The model under review builds one solid part; all positions refer to its coordinate system, in mm. A direction names the side the tool comes from. Coordinates: 2 decimals unless noted, no trailing zeros. Order: outer loops, then holes, each group sorted by start corner. A loop starts at its lowest first (then second) coordinate and runs counter-clockwise, first axis right, second up. Notation, with made-up numbers: M -31.75,26.5 L -1.75,26.5 A19 ccw -1.75,55.5 Z; hole C -11.75,2.25 d1. An arc over 180 degrees is marked long. Answer as CSV lines item,"result". Start each with the question number.
Q1. Machinability: for faces 5 (the face through (-17.691, -13, 6)), 6 (the face through (1, 0, 2)), which of the approach directions +Z, -Z, +X, -X, +Y, -Y give a long, thin tool a straight path to every point of the face, cutting with its end or side? Answer none if there is none.
Q2. Consider section B-B on z = 25. Write out the cut boundary in (x, y), and give its area (3 significant figures).
Q3. The part is to be moulded in two halves that separate along X. For faces 1 (the face through (-3, -13, -20.358)), 2 (the face through (1, -13, -42.939)), 3 (the face through (-46.495, -13, 0)), 4 (the face through (36.716, -13, 25)), say which applies: +X half, -X half, draft (parallel to the pull), parting line (faces both ways), or undercut.
Q4. Consider section D-D on x = -27. Write out the cut boundary in (y, z), and give its area (3 significant figures).
Q5. Consider section C-C on y = -21. Write out the cut boundary in (x, z), and give its area (3 significant figures).
Q6. Wall thickness on L1, parallel to Z at x = 17, y = -19.5; L2, parallel to Z at x = 29.5, y = -4.75; L3, parallel to X at y = -10.75, z = 26: over which ranges is each line inside the solid? List them lowest first. Write a range as [from, to].
Q7. Consider section A-A on x = -5. Write out the cut boundary in (y, z), and give its area (3 significant figures).
Q8. For P1, Ø1, axis at x = -13, z = -11.5, coming from the +Y side, flat-tipped, find the tip position at first contact; note if it passes through.
from build123d import *

# Parameters (mm, degrees)
F0_W     = 96.367601
F0_H     = 87.655403
F1_DEPTH = 25.4
F4_DEPTH = 25.4


with BuildPart() as f1:
    # F0 (on Front) → F1 (new body)
    with BuildSketch(Plane.XZ):
        with Locations((1.689101, 0.889)):
            Rectangle(F0_W, F0_H)
    extrude(amount=F1_DEPTH)

    # F3 (on face) + F2 (on face) → F4 (cut)
    with BuildSketch(Plane.XZ.offset(25.4)):
        Polygon((36.715697, 12.179299), (36.715697, 37.604701), (-29.248102, 37.604701), (-29.248102, -8.6233), (22.1361, -8.6233), (22.1361, -20.358101), (-29.248102, -20.358101), (-29.248102, -34.048699), (36.715697, -34.048699), (36.715697, 0), (-17.6911, 0), (-17.6911, 12.179299), align=None)
    with BuildSketch(Plane.XZ.offset(25.4)):
        Polygon((36.715697, 37.604701), (-29.248102, 37.604701), (-29.248102, -8.6233), (22.1361, -8.6233), (22.1361, -20.358101), (-29.248102, -20.358101), (-29.248102, -34.048699), (36.715697, -34.048699), (36.715697, 0), (-17.6911, 0), (-17.6911, 12.179299), (36.715697, 12.179299), align=None)
    extrude(amount=-F4_DEPTH, mode=Mode.SUBTRACT)


solid = f1.part
Evaluation:
1,face 5,"+Y, -Y"
1,face 6,"+Z, -Z, +X, -X, +Y"
2,outline,"M -46.49,-25.4 L -29.25,-25.4 L -29.25,0 L -46.49,0 Z; M 36.72,-25.4 L 49.87,-25.4 L 49.87,0 L 36.72,0 Z"
2,area,"772 mm²"
3,face 1,"undercut"
3,face 2,"draft"
3,face 3,"-X half"
3,face 4,"undercut"
4,outline,"M -25.4,-42.94 L 0,-42.94 L 0,-34.05 L -25.4,-34.05 Z; M -25.4,-20.36 L 0,-20.36 L 0,-8.62 L -25.4,-8.62 Z; M -25.4,37.6 L 0,37.6 L 0,44.72 L -25.4,44.72 Z"
4,area,"705 mm²"
5,outline,"M -46.49,-42.94 L 49.87,-42.94 L 49.87,44.72 L -46.49,44.72 Z; hole M -29.25,-34.05 L 36.72,-34.05 L 36.72,0 L -17.69,0 L -17.69,12.18 L 36.72,12.18 L 36.72,37.6 L -29.25,37.6 L -29.25,-8.62 L 22.14,-8.62 L 22.14,-20.36 L -29.25,-20.36 Z"
5,area,"4,990 mm²"
6,L1,"z = [-42.94, -34.05], [-20.36, -8.62], [0, 12.18], [37.6, 44.72]"
6,L2,"z = [-42.94, -34.05], [0, 12.18], [37.6, 44.72]"
6,L3,"x = [-46.49, -29.25], [36.72, 49.87]"
7,outline,"M -25.4,-42.94 L 0,-42.94 L 0,-34.05 L -25.4,-34.05 Z; M -25.4,-20.36 L 0,-20.36 L 0,-8.62 L -25.4,-8.62 Z; M -25.4,0 L 0,0 L 0,12.18 L -25.4,12.18 Z; M -25.4,37.6 L 0,37.6 L 0,44.72 L -25.4,44.72 Z"
7,area,"1,010 mm²"
8,P1,"stops at y = 0"
